from build123d import *

# Parameters (mm, degrees)
SKETCH1_R               = 1.6
BOSS_EXTRUDE1_DEPTH     = 4.2
SKETCH2_W               = 15
SKETCH2_H               = 15
BOSS_EXTRUDE2_DEPTH     = 2
FILLET1_R               = 3
SKETCH3_R               = 1.6
CUT_EXTRUDE1_DEPTH      = 5.2
CUT_EXTRUDE1_DEPTH_BACK = 3


with BuildPart() as part:
    # Sketch1 → Boss-Extrude1 (new body)
    with BuildSketch(Plane(origin=(0, 0, 0), x_dir=(1, 0, 0), z_dir=(0, 1, 0))):
        with BuildLine():
            Line((-3, -2), (-3, 2))
            ThreePointArc((-3, 2), (0, 5), (3, 2))
            Line((3, 2), (3, -2))
            ThreePointArc((3, -2), (0, -5), (-3, -2))
        make_face()
        Circle(SKETCH1_R, mode=Mode.SUBTRACT)
    extrude(amount=BOSS_EXTRUDE1_DEPTH)

    # Sketch2 → Boss-Extrude2 (add)
    with BuildSketch(Plane.XZ):
        Rectangle(SKETCH2_W, SKETCH2_H)
    extrude(amount=BOSS_EXTRUDE2_DEPTH)

    # Fillet1
    fillet1_edges = [part.edges().sort_by_distance(p)[0] for p in [
        (-7.5, -1, 7.5),
        (-7.5, -1, -7.5),
        (7.5, -1, -7.5),
        (7.5, -1, 7.5),
    ]]
    fillet(fillet1_edges, radius=FILLET1_R)

    # Sketch3 → Cut-Extrude1 (cut, two sides)
    with BuildSketch(Plane(origin=(0, 0, 0), x_dir=(1, 0, 0), z_dir=(0, 1, 0))) as cut_extrude1_sk:
        Circle(SKETCH3_R)
    extrude(amount=CUT_EXTRUDE1_DEPTH, mode=Mode.SUBTRACT)
    extrude(cut_extrude1_sk.sketch, amount=-CUT_EXTRUDE1_DEPTH_BACK, mode=Mode.SUBTRACT)


solid = part.part
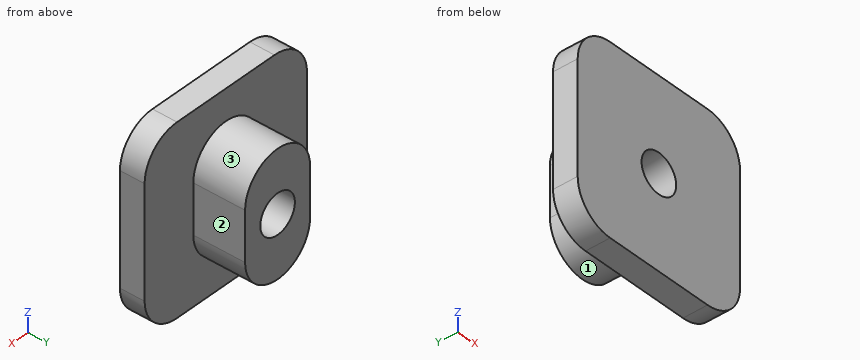
For this review, take the finished solid that the model builds, in its own axes (mm). Face numbers are marked on the shaded views. A direction names the side the tool comes from. Coordinates: 2 decimals unless noted, no trailing zeros. Loops run counter-clockwise (first coordinate to the right, second up) from the corner with the lowest first, then second, coordinate; pieces in that order, holes last. Notation, with made-up numbers: (-22.5, 1) -> (-2.5, 1) arc R19 cw to (-2.5, 17) -> close; hole circle Ø10 at (-39.75, 67). An arc over 180 degrees is marked (long way). Write each question's results on one line, items separated by ' | '.
Q1. Add section D-D, the plane x = 2.5. State the section outline as (y, z) points.
Taken from the geometry:
outline: (-2, -7.5) -> (0, -7.5) -> (0, -3.66) -> (4.2, -3.66) -> (4.2, 3.66) -> (0, 3.66) -> (0, 7.5) -> (-2, 7.5) -> close
Q2. Add section A-A, the plane y = -1. State the section outline as (x, z) points, then the cut area to 3 significant figures.
Taken from the geometry:
outline: (-7.5, -4.5) arc R3 ccw to (-4.5, -7.5) -> (4.5, -7.5) arc R3 ccw to (7.5, -4.5) -> (7.5, 4.5) arc R3 ccw to (4.5, 7.5) -> (-4.5, 7.5) arc R3 ccw to (-7.5, 4.5) -> close; hole circle Ø3.2 at (0, 0) | area: 209 mm²
Q3. Machinability: for the marked faces 1, 2 and 3, which of the approach directions +Z, -Z, +X, -X, +Y, -Y give a long, thin tool a straight path to every point of the face, cutting with its end or side? Answer none if there is none.
Taken from the geometry:
face 1: -Z, +Y | face 2: +Z, -Z, +X, +Y | face 3: +Z, +Y
Q4. Add section B-B, the plane x = 0. State the section outline as (y, z) points.
Taken from the geometry:
outline: (-2, -7.5) -> (0, -7.5) -> (0, -5) -> (4.2, -5) -> (4.2, -1.6) -> (-2, -1.6) -> close; (-2, 1.6) -> (4.2, 1.6) -> (4.2, 5) -> (0, 5) -> (0, 7.5) -> (-2, 7.5) -> close
Q5. To check wall thickness, follow line 1 along X through (y, z) = (1.45, 0); line 2 along Z through (x, y) = (0, -1). State the ranges of each line that lie inside material, in increasing order. Write a range as [from, to].
Taken from the geometry:
line 1: [-3, -1.6], [1.6, 3] | line 2: [-7.5, -1.6], [1.6, 7.5]
Q6. Add section C-C, the plane z = 0. State the section outline as (x, y) points.
Taken from the geometry:
outline: (-7.5, -2) -> (-1.6, -2) -> (-1.6, 4.2) -> (-3, 4.2) -> (-3, 0) -> (-7.5, 0) -> close; (1.6, -2) -> (7.5, -2) -> (7.5, 0) -> (3, 0) -> (3, 4.2) -> (1.6, 4.2) -> close
Q7. For pin 1 Ø1 at (y, z) = (2.5, 1.5) entering from +X, flat-tipped, find the tip position at first contact; note if it passes through.
Taken from the geometry:
pin 1: x = 3
